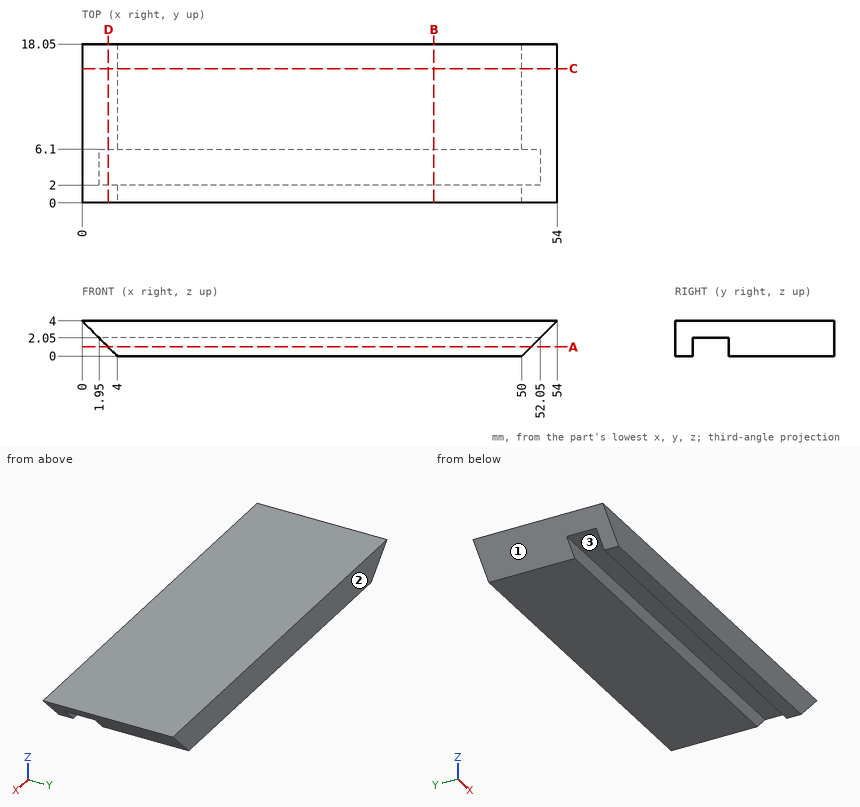
Here's the drawing with two shaded views (mm, measured from the low corner). I have some questions. Coordinates: 2 decimals unless noted, no trailing zeros. Write each loop counter-clockwise with the first axis right and the second up, starting at its lowest first coordinate (ties: lowest second). Pieces come first, ordered by that corner, then holes. Notation, with made-up numbers: (34.25, 2) -> (68.25, 2) arc R20 cw to (68.25, 37) -> close; hole circle Ø3 at (32, -11.75). An arc over 180 degrees is marked (long way). Answer as CSV lines item,"result".
1) If we section it at A-A on z = 1.05: Please give me the cut outline in (x, y), then the cut area to 3 significant figures.
Check result:
outline,"(2.95, 0) -> (51.05, 0) -> (51.05, 2) -> (2.95, 2) -> close; (2.95, 6.1) -> (51.05, 6.1) -> (51.05, 18.05) -> (2.95, 18.05) -> close"
area,"671 mm²"
2) If we section it at C-C on y = 15.25: Please give me the cut outline in (x, z).
Check result:
outline,"(0, 4) -> (4, 0) -> (50, 0) -> (54, 4) -> close"
3) If I drill on line 1 (Y direction, x = 19, z = 2); line 2 (Z direction, x = 35, y = 3.75); line 3 (X direction, y = 13, z = 3), over which ranges is the centre line in solid material (lowest first)? Write a range as from..to.
Check result:
line 1,"0..2, 6.1..18.05"
line 2,"2.05..4"
line 3,"1..53"
4) If we section it at B-B on x = 40: Please give me the cut outline in (y, z).
Check result:
outline,"(0, 0) -> (2, 0) -> (2, 2.05) -> (6.1, 2.05) -> (6.1, 0) -> (18.05, 0) -> (18.05, 4) -> (0, 4) -> close"
5) If we section it at D-D on x = 3: Please give me the cut outline in (y, z).
Check result:
outline,"(0, 1) -> (2, 1) -> (2, 2.05) -> (6.1, 2.05) -> (6.1, 1) -> (18.05, 1) -> (18.05, 4) -> (0, 4) -> close"
6) Will these pins go through, and if not, where does the flat tip stop? P1, Ø3.5, axis at x = 23, y = 4, coming from the -Z side; P2, Ø2, axis at y = 10, z = 1, coming from the +X side.
Check result:
P1,"z = 2.05"
P2,"x = 52"
7) If we mould it in two halves opening along Y, with no side actions, what happens to the marked faces 1, 2 and 3? For each: +Y half, -Y half, draft (parallel to the pull), parting line (faces both ways), or undercut.
Check result:
face 1,"draft"
face 2,"+Y half"
face 3,"undercut"
